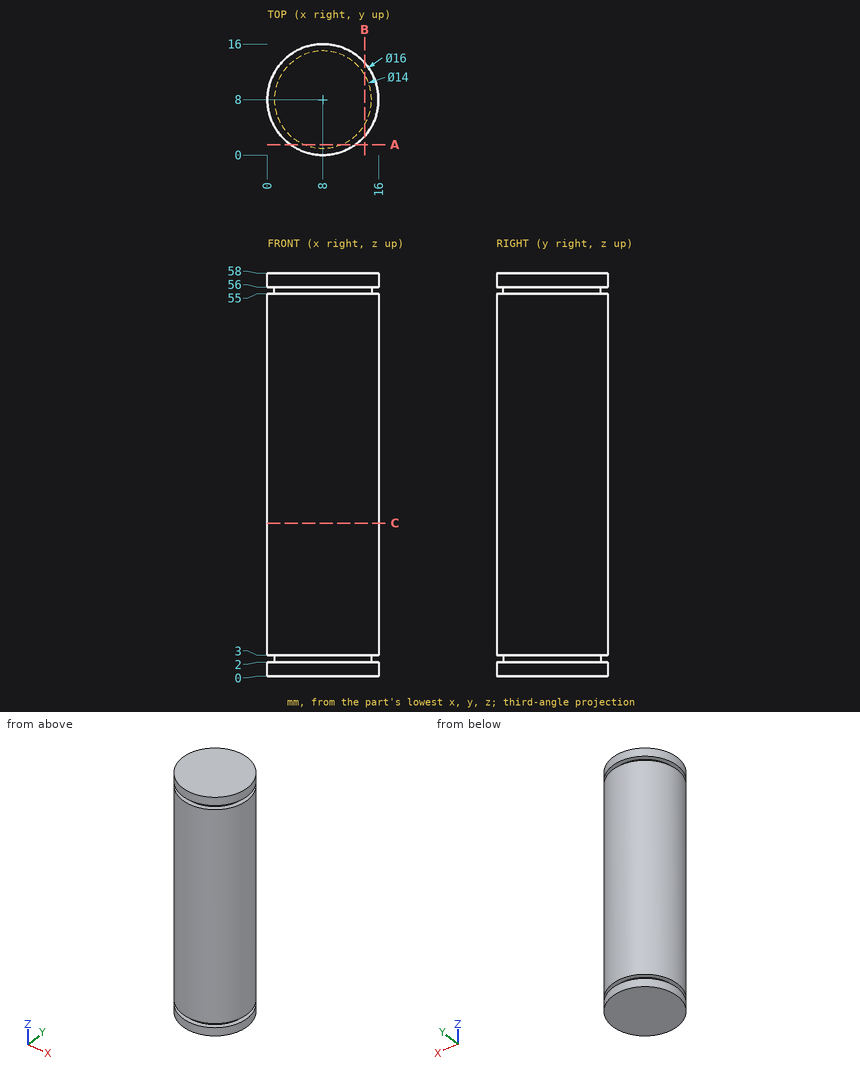
Check sheet for the drawn part. Datum: minimum x, y, z corner. Units: mm. Give positions to 0.01 mm unless a question says otherwise; leave off trailing zeros. Write each loop counter-clockwise with the first axis right and the second up, starting at its lowest first coordinate (ties: lowest second). Pieces come first, ordered by that corner, then holes. Notation, with made-up numbers: M 59,51 L 74,51 A25 cw 74,76 Z; hole C 81.5,12.5 d4. An arc over 180 degrees is marked long. Write item = value, one per line.
(1) Material ranges on line 1 (Z direction, x = 14.75, y = 10.75); line 2 (Y direction, x = 7.75, z = 41.5); line 3 (X direction, y = 15.25, z = 10), recorded low to high.
Found:
line_1 = 0 to 2, 3 to 55, 56 to 58
line_2 = 0 to 16
line_3 = 4.62 to 11.38
(2) Go/stop test with flat-tipped pins: pin 1 Ø2 at (y, z) = (11, 37) entering from +X; pin 2 Ø3 at (x, y) = (12, 9.5) entering from -Z; pin 3 Ø4 at (x, z) = (13.5, 37) entering from +Y. Record where each tip stops, or that it passes through.
Found:
pin_1 = 15.75
pin_2 = 0
pin_3 = 15.19
(3) Sectioned sample at C-C (z = 22). Record the cut outline in (x, y), then the cut area to 3 significant figures.
Found:
outline = C 8,8 d16
area = 201 mm2
(4) Sectioned sample at B-B (x = 14). Record the cut outline in (y, z), then the cut area to 3 significant figures.
Found:
outline = M 2.71,0 L 13.29,0 L 13.29,2 L 11.61,2 L 11.61,3 L 13.29,3 L 13.29,55 L 11.61,55 L 11.61,56 L 13.29,56 L 13.29,58 L 2.71,58 L 2.71,56 L 4.39,56 L 4.39,55 L 2.71,55 L 2.71,3 L 4.39,3 L 4.39,2 L 2.71,2 Z
area = 607 mm2
(5) Sectioned sample at A-A (y = 1.5). Record the cut outline in (x, z).
Found:
outline = M 3.34,0 L 12.66,0 L 12.66,2 L 10.6,2 L 10.6,3 L 12.66,3 L 12.66,55 L 10.6,55 L 10.6,56 L 12.66,56 L 12.66,58 L 3.34,58 L 3.34,56 L 5.4,56 L 5.4,55 L 3.34,55 L 3.34,3 L 5.4,3 L 5.4,2 L 3.34,2 Z
